Geometry check sheet. Reference: the model listing, model coordinates, mm. Face numbers are marked on the shaded views. A direction names the side the tool comes from. Round coordinates to 2 decimals unless told otherwise and drop trailing zeros. Order: outer loops, then holes, each group sorted by start corner. A loop starts at its lowest first (then second) coordinate and runs counter-clockwise, first axis right, second up.
(1) Cross-section at A-A on z = -39. Enter the section's corners in (x, y), and give its area (3 significant figures).
(2) Set-up check for the marked faces 4 and 5: record each of +Z, -Z, +X, -X, +Y, -Y from which the full face is reachable in a straight line by a thin tool's end or side.
(3) Cross-section at B-B on x = 11. Enter the section's corners in (y, z), and give its area (3 significant figures).
(4) Cross-section at C-C on z = -19. Enter the section's corners in (x, y).
(5) Draft check along X on the marked faces 1, 2 and 3. Enter one of: pulls with the +X half, pulls with the -X half, needs draft (parallel to the pull), parting line crosses it, or undercut.
(6) Cross-section at D-D on x = -15.5. Enter the section's corners in (y, z).
(7) Thickness scan on L1, parallel to X at y = 0.5, z = -2.5; L2, parallel to X at y = -3.5, z = -14.5; L3, parallel to Y at x = 11, z = -41. Record the ranges inside material, lowest first.
(8) Gauge pin test, flat ends, axial feed: P1, Ø0.9, axis at y = 0.5, z = -4, coming from the +X side; P2, Ø10.5, axis at x = 12.5, z = -13.5, coming from the -Y side; P3, Ø9, axis at x = 11.5, y = -0.5, coming from the -Z side; P4, Ø4, axis at y = 0, z = -22, coming from the -X side. Record the tip position at first contact, or that the pin passes through.
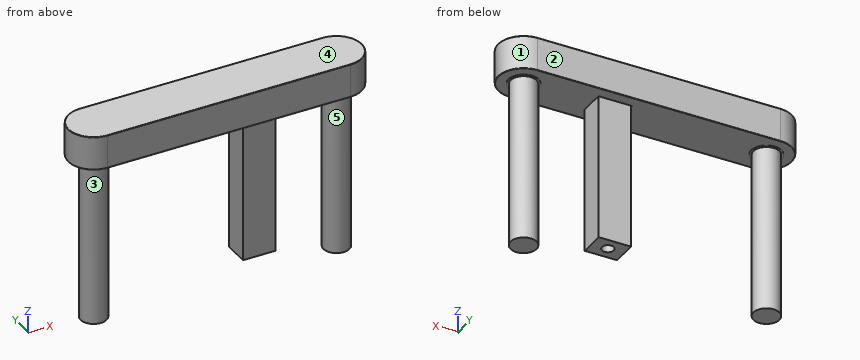
from build123d import *

# Parameters (mm, degrees)
SKETCH1_R           = 4
BOSS_EXTRUDE1_DEPTH = 5
FILLET2_R           = 0.15
SKETCH2_W           = 10
SKETCH2_H           = 7.9994
CUT_EXTRUDE1_DEPTH  = 3
SKETCH3_R           = 1.75
CUT_EXTRUDE2_DEPTH  = 45.69339996
SKETCH4_R           = 4.15
BOSS_EXTRUDE2_DEPTH = 10
SKETCH5_R           = 4.5
BOSS_EXTRUDE3_DEPTH = 0.1
SKETCH6_R           = 3.85
BOSS_EXTRUDE4_DEPTH = 49.5
SKETCH9_W           = 9.6
SKETCH9_H           = 7.5994
BOSS_EXTRUDE5_DEPTH = 53.1
SKETCH10_R          = 1.75
CUT_EXTRUDE3_DEPTH  = 10


with BuildPart() as part:
    # Sketch1 → Boss-Extrude1 (new, symmetric)
    with BuildSketch(Plane.XY):
        with BuildLine():
            Line((-35.999998845, 7.5), (35.999998845, 7.5))
            ThreePointArc((35.999998845, 7.5), (43.5, 0), (35.999998845, -7.5))
            Line((35.999998845, -7.5), (-35.999998845, -7.5))
            ThreePointArc((-35.999998845, -7.5), (-43.5, 0), (-35.999998845, 7.5))
        make_face()
        with Locations((-36, 0)):
            Circle(SKETCH1_R, mode=Mode.SUBTRACT)
        with Locations((36, 0)):
            Circle(SKETCH1_R, mode=Mode.SUBTRACT)
    extrude(amount=BOSS_EXTRUDE1_DEPTH, both=True)

    # Fillet2
    fillet2_edges = [part.edges().sort_by_distance(p)[0] for p in [
        (-40, 0, -5),
        (-40, 0, 5),
        (-43.5, 0, 5),
        (32, 0, -5),
        (32, 0, 5),
        (0, -7.5, 5),
        (43.5, 0, 5),
        (0, -7.5, -5),
        (-43.5, 0, -5),
        (0, 7.5, -5),
        (43.5, 0, -5),
        (0, 7.5, 5),
    ]]
    fillet(fillet2_edges, radius=FILLET2_R)

    # Sketch2 → Cut-Extrude1 (cut)
    with BuildSketch(Plane(origin=(0, 0, -5), x_dir=(-1, 0, 0), z_dir=(0, 0, -1))):
        with Locations((-11, 0.0003)):
            Rectangle(SKETCH2_W, SKETCH2_H)
    extrude(amount=-CUT_EXTRUDE1_DEPTH, mode=Mode.SUBTRACT)

    # Sketch3 → Cut-Extrude2 (cut, through all)
    with BuildSketch(Plane(origin=(0, 0, -2), x_dir=(-1, 0, 0), z_dir=(0, 0, -1))):
        with Locations((-11, 0.0003)):
            Circle(SKETCH3_R)
    extrude(amount=-CUT_EXTRUDE2_DEPTH, mode=Mode.SUBTRACT)

    # Sketch4 → Boss-Extrude2 (add)
    with BuildSketch(Plane.XY.offset(5)):
        with Locations((36, 0)):
            Circle(SKETCH4_R)
        with Locations((-36, 0)):
            Circle(SKETCH4_R)
    extrude(amount=-BOSS_EXTRUDE2_DEPTH)

    # Sketch5 → Boss-Extrude3 (add)
    with BuildSketch(Plane(origin=(0, 0, -5), x_dir=(-1, 0, 0), z_dir=(0, 0, -1))):
        with Locations(Location((36, 0, 0), (0, 0, 180))):
            Circle(SKETCH5_R)
        with Locations(Location((-36, 0, 0), (0, 0, 180))):
            Circle(SKETCH5_R)
    extrude(amount=BOSS_EXTRUDE3_DEPTH)

    # Sketch6 → Boss-Extrude4 (add)
    with BuildSketch(Plane(origin=(0, 0, -5.1), x_dir=(-1, 0, 0), z_dir=(0, 0, -1))):
        with Locations((-36, 0)):
            Circle(SKETCH6_R)
        with Locations((36, 0)):
            Circle(SKETCH6_R)
    extrude(amount=BOSS_EXTRUDE4_DEPTH)

    # Sketch9 → Boss-Extrude5 (add)
    with BuildSketch(Plane.XY.offset(5)):
        with Locations((11, 0.0003)):
            Rectangle(SKETCH9_W, SKETCH9_H)
    extrude(amount=-BOSS_EXTRUDE5_DEPTH)

    # Sketch10 → Cut-Extrude3 (cut)
    with BuildSketch(Plane(origin=(0, 0, -48.1), x_dir=(-1, 0, 0), z_dir=(0, 0, -1))):
        with Locations((-11, 0.0003)):
            Circle(SKETCH10_R)
    extrude(amount=-CUT_EXTRUDE3_DEPTH, mode=Mode.SUBTRACT)


solid = part.part
Found:
1. outline: circle Ø7.7 at (-36, 0); (6.2, -3.8) - (15.8, -3.8) - (15.8, 3.8) - (6.2, 3.8) - close; circle Ø7.7 at (36, 0); hole circle Ø3.5 at (11, 0)
1. area: 156 mm2
2. face 4: +Z, +X, -X, +Y, -Y
2. face 5: -Z
3. outline: (-7.5, -4.85) arc R0.15 ccw to (-7.35, -5) - (-4, -5) - (-4, -2) - (-3.8, -2) - (-3.8, -48.1) - (-1.75, -48.1) - (-1.75, -38.1) - (1.75, -38.1) - (1.75, -48.1) - (3.8, -48.1) - (3.8, -2) - (4, -2) - (4, -5) - (7.35, -5) arc R0.15 ccw to (7.5, -4.85) - (7.5, 4.85) arc R0.15 ccw to (7.35, 5) - (-7.35, 5) arc R0.15 ccw to (-7.5, 4.85) - close
3. area: 441 mm2
4. outline: circle Ø7.7 at (-36, 0); (6.2, -3.8) - (15.8, -3.8) - (15.8, 3.8) - (6.2, 3.8) - close; circle Ø7.7 at (36, 0)
5. face 1: pulls with the +X half
5. face 2: needs draft
5. face 3: undercut
6. outline: (-7.5, -4.85) arc R0.15 ccw to (-7.35, -5) - (7.35, -5) arc R0.15 ccw to (7.5, -4.85) - (7.5, 4.85) arc R0.15 ccw to (7.35, 5) - (-7.35, 5) arc R0.15 ccw to (-7.5, 4.85) - close
7. L1: x = -43.48 to 6, 6.2 to 15.8, 16 to 43.48
7. L2: x = -37.6 to -34.4, 6.2 to 15.8, 34.4 to 37.6
7. L3: y = -3.8 to -1.75, 1.75 to 3.8
8. P1: stops at x = 43.5
8. P2: stops at y = -3.8
8. P3: stops at z = -48.1
8. P4: stops at x = -39.85
